Source: CAD feature listing. Evaluate the final solid. Frame: model axes, mm. Coordinates: 2 decimals unless noted, no trailing zeros. Loops run counter-clockwise (first coordinate to the right, second up) from the corner with the lowest first, then second, coordinate; pieces in that order, holes last. Notation, with made-up numbers: (13, 23) - (38, 23) arc R17 cw to (38, 56) - close; hole circle Ø6 at (32.5, 14.25). An arc over 180 degrees is marked (long way). Use one line per item in the form item = value. Start each with the question number.
from build123d import *

# Parameters (mm, degrees)
SKETCH1_R           = 3.1
SKETCH1_R_2         = 3.175
SKETCH1_R_3         = 15.875
BOSS_EXTRUDE1_DEPTH = 1.5875
FILLET1_R           = 2


with BuildPart() as part:
    # Sketch1 → Boss-Extrude1 (new, symmetric)
    with BuildSketch(Plane.XY):
        with BuildLine():
            Line((-15.202382741, 38.1), (-123.202382741, 38.1))
            Line((-123.202382741, 38.1), (-123.202382741, -38.1))
            Line((-123.202382741, -38.1), (-15.202382741, -38.1))
            ThreePointArc((-15.202382741, -38.1), (0, -41.021), (15.202382741, -38.1))
            Line((15.202382741, -38.1), (123.202382741, -38.1))
            Line((123.202382741, -38.1), (123.202382741, 38.1))
            Line((123.202382741, 38.1), (15.202382741, 38.1))
            ThreePointArc((15.202382741, 38.1), (0, 41.021), (-15.202382741, 38.1))
        make_face()
        with Locations((-111.202382741, 24)):
            Circle(SKETCH1_R, mode=Mode.SUBTRACT)
        with Locations((-63.202382741, 24)):
            Circle(SKETCH1_R, mode=Mode.SUBTRACT)
        with Locations((-63.202382741, -24)):
            Circle(SKETCH1_R, mode=Mode.SUBTRACT)
        with Locations((-111.202382741, -24)):
            Circle(SKETCH1_R, mode=Mode.SUBTRACT)
        with Locations((111.202382741, -24)):
            Circle(SKETCH1_R, mode=Mode.SUBTRACT)
        with Locations((63.202382741, -24)):
            Circle(SKETCH1_R, mode=Mode.SUBTRACT)
        with Locations(Location((63.202382741, 24, 0), (0, 0, 180))):
            Circle(SKETCH1_R, mode=Mode.SUBTRACT)
        with Locations((111.202382741, 24)):
            Circle(SKETCH1_R, mode=Mode.SUBTRACT)
        with Locations((0, 34.925)):
            Circle(SKETCH1_R_2, mode=Mode.SUBTRACT)
        with Locations((30.245937227, 17.4625)):
            Circle(SKETCH1_R_2, mode=Mode.SUBTRACT)
        with Locations((30.245937227, -17.4625)):
            Circle(SKETCH1_R_2, mode=Mode.SUBTRACT)
        with Locations((0, -34.925)):
            Circle(SKETCH1_R_2, mode=Mode.SUBTRACT)
        with Locations((-30.245937227, -17.4625)):
            Circle(SKETCH1_R_2, mode=Mode.SUBTRACT)
        with Locations((-30.245937227, 17.4625)):
            Circle(SKETCH1_R_2, mode=Mode.SUBTRACT)
        Circle(SKETCH1_R_3, mode=Mode.SUBTRACT)
    extrude(amount=BOSS_EXTRUDE1_DEPTH, both=True)

    # Fillet1
    fillet1_edges = [part.edges().sort_by_distance(p)[0] for p in [
        (-15.202382741, 38.1, 0),
        (-15.202382741, -38.1, 0),
        (15.202382741, -38.1, 0),
        (15.202382741, 38.1, 0),
    ]]
    fillet(fillet1_edges, radius=FILLET1_R)


solid = part.part
(1) Mould query, pull axis X, two halves, no side actions, for faces 1 (the face through (31.95, 20.14, -0.02)), 2 (the face through (-2, 19, 1.588)), 3 (the face through (-65.66, -25.89, -0.02)). Classes: +X half, -X half, draft (parallel to the pull), parting line (faces both ways), or undercut.
(2) Contact query for flat-ended pins moving along their axis: pin 1 (8.5 mm diameter, centred on x = -30.25, y = 17.46, fed in from -Z); pin 2 (5.5 mm diameter, centred on x = -30.25, y = -17.46, fed in from -Z); pin 3 (1 mm diameter, centred on x = 85, z = 0.5, fed in from +Y); pin 4 (1 mm diameter, centred on x = -44, z = -0.5, fed in from -Y). Output: stop coordinate, or through.
(3) Material intervals for line 1 (Y direction, x = 30.5, z = 0.2); line 2 (Y direction, x = -0.5, z = -0.3); line 3 (X direction, y = -0.5, z = 0.05), sorted ascending.
(4) Cut plane C-C, the plane y = -24. Output: boundary loops of the cut face in (x, z).
(5) Cut plane A-A, the plane x = 0. State how many separate pieces and enclosed holes the cut face has, plus the area to 3 significant figures.
(6) Cut plane B-B, the plane y = 0. Output: boundary loops of the cut face in (x, z) (1 decimal).
Recorded:
q1.face_1 = undercut
q1.face_2 = draft
q1.face_3 = undercut
q2.pin_1 = -1.59
q2.pin_2 = through
q2.pin_3 = 38.1
q2.pin_4 = -38.1
q3.line_1 = -38.1 to -20.63, -14.3 to 14.3, 20.63 to 38.1
q3.line_2 = -41.02 to -38.06, -31.79 to -15.87, 15.87 to 31.79, 38.06 to 41.02
q3.line_3 = -123.2 to -15.87, 15.87 to 123.2
q4.outline = (-123.2, -1.59) - (-114.3, -1.59) - (-114.3, 1.59) - (-123.2, 1.59) - close; (-108.1, -1.59) - (-66.3, -1.59) - (-66.3, 1.59) - (-108.1, 1.59) - close; (-60.1, -1.59) - (60.1, -1.59) - (60.1, 1.59) - (-60.1, 1.59) - close; (66.3, -1.59) - (108.1, -1.59) - (108.1, 1.59) - (66.3, 1.59) - close; (114.3, -1.59) - (123.2, -1.59) - (123.2, 1.59) - (114.3, 1.59) - close
q5.separate_pieces = 4
q5.enclosed_holes = 0
q5.area = 119 mm²
q6.outline = (-123.2, -1.6) - (-15.9, -1.6) - (-15.9, 1.6) - (-123.2, 1.6) - close; (15.9, -1.6) - (123.2, -1.6) - (123.2, 1.6) - (15.9, 1.6) - close
